```python
from build123d import *

# Parameters (mm, degrees)
F1_DEPTH = 241.3
F2_T     = -2.54


with BuildPart() as f1:
    # F0 (on Right) → F1 (new body, symmetric)
    with BuildSketch(Plane.YZ):
        Polygon((-254, 0), (0, 0), (0, 254), align=None)
    extrude(amount=F1_DEPTH, both=True)

    # F2
    f2_openings = [f1.faces().sort_by_distance(p)[0] for p in [
        (0, 0, 127),
        (0, -127, 0),
    ]]
    offset(amount=F2_T, openings=f2_openings)


solid = f1.part
```
Geometry check sheet. Reference: the model listing, model coordinates, mm. A direction names the side the tool comes from. Round coordinates to 2 decimals unless told otherwise and drop trailing zeros. Order: outer loops, then holes, each group sorted by start corner. A loop starts at its lowest first (then second) coordinate and runs counter-clockwise, first axis right, second up. Notation, with made-up numbers: (31, 76.25) -> (82, 76.25) arc R23 cw to (82, 104.25) -> close; hole circle Ø5 at (40, -37.5). An arc over 180 degrees is marked (long way). Return JSON: item names as keys, results as strings. Group by question number.
Q1. Section check A-A, the plane z = 236.5. Record the boundary of the cut face in (x, y).
Q2. Tool access check on faces 4 (the flat face through (238.76, -71, 71)), 5 (the flat face through (-241.3, -72, 72)). Record the directions out of +Z, -Z, +X, -X, +Y, -Y that give a thin tool (end or side, any length) a straight path to the whole face; none if there is none.
Q3. Gauge pin test, flat ends, axial feed: pin 1 (5 mm diameter, centred on x = 91, y = -135.5, fed in from +Z); pin 2 (10 mm diameter, centred on x = 93, y = -90.5, fed in from +Z); pin 3 (5 mm diameter, centred on x = -116.5, y = -63, fed in from -Z). Record the tip position at first contact, or that the pin passes through.
Q4. Section check B-B, the plane y = -191.5. Record the boundary of the cut face in (x, z), plus the area to 3 significant figures.
Q5. Material ranges on probe 1 along X at (y, z) = (-54.5, 29.5); probe 2 along Y at (x, z) = (-170, 25.5); probe 3 along Y at (x, z) = (-59.5, 106), recorded low to high. Write a range as from..to.
Q6. Section check C-C, the plane x = 75. Record the boundary of the cut face in (y, z), plus the area to 3 significant figures.
Q7. Release check for a two-part mould opening along X. For faces 1 (the flat face through (241.3, -72, 72)), 2 (the flat face through (-238.76, -71, 71)), 3 (the flat face through (3, -125, 129)) record: released by +X, released by -X, zero draft, split by the parting line, or undercut.
Numbers:
{
 "1": {"outline": "(-241.3, -17.5) -> (241.3, -17.5) -> (241.3, 0) -> (238.76, 0) -> (238.76, -13.91) -> (-238.76, -13.91) -> (-238.76, 0) -> (-241.3, 0) -> close"},
 "2": {"face 4": "-Z, +Y", "face 5": "+Z, -Z, -X, +Y, -Y"},
 "3": {"pin 1": "z = 121", "pin 2": "z = 168.5", "pin 3": "z = 184.91"},
 "4": {"outline": "(-241.3, 0) -> (-238.76, 0) -> (-238.76, 58.91) -> (238.76, 58.91) -> (238.76, 0) -> (241.3, 0) -> (241.3, 62.5) -> (-241.3, 62.5) -> close", "area": "2,030 mm^2"},
 "5": {"probe 1": "-241.3..-238.76, 238.76..241.3", "probe 2": "-228.5..-224.91", "probe 3": "-148..-144.41"},
 "6": {"outline": "(-254, 0) -> (-250.41, 0) -> (0, 250.41) -> (0, 254) -> close", "area": "906 mm^2"},
 "7": {"face 1": "released by +X", "face 2": "undercut", "face 3": "zero draft"}
}
